CAD build for the part. Positions are in the model's coordinates, mm. A direction names the side the tool comes from. Round coordinates to 2 decimals unless told otherwise and drop trailing zeros. Order: outer loops, then holes, each group sorted by start corner. A loop starts at its lowest first (then second) coordinate and runs counter-clockwise, first axis right, second up. Notation, with made-up numbers: (27.5, -30) -> (52.5, -30) arc R16 ccw to (52.5, -24) -> close; hole circle Ø11 at (41.5, -6). An arc over 180 degrees is marked (long way). Return JSON: item names as keys, results as strings. Group by question number.
Q1. Flat gauge pins, fed straight in: pin 1 (1 mm diameter, centred on x = -29, y = -14.5, fed in from +Z); pin 2 (3 mm diameter, centred on x = -33, z = 2, fed in from -Y); pin 3 (3 mm diameter, centred on x = -46.5, y = -6.5, fed in from +Z). Where does each tip first touch, or does it go through?
Q2. Cut at A-A (z = 0). Write the cut outline in (x, y).
Q3. Mould opens along Z. For faces 4 (the flat face through (-70.245, -8.8, 9)), 5 (the cylindrical face through (-1.824, -60.029, -23.647)), 6 (the conical face through (10.1, 11.2, 36)) say: +Z half, -Z half, draft (parallel to the pull), parting line (faces both ways), or undercut.
Q4. Which spindle directions (+Z, -Z, +X, -X, +Y, -Y) get a long thin tool onto all of the face, cutting with end or side? Do faces 1 (the flat face through (-25.245, -36, 46)), 2 (the cylindrical face through (-1.824, 9.745, 23.647)), 3 (the flat face through (-42, -4.642, 0)). Say none if no direction does.
Q5. Probe line 1 along Y through (x, z) = (-50, 0); line 2 along X through (y, z) = (8, 7); line 3 along Y through (x, z) = (-15, 1). List the from-to ranges inside material, lowest first.
Q6. Cut at B-B (x = -11). Write the cut outline in (y, z).
Q7. Cut at C-C (x = -44.5). Write the cut outline in (y, z).
from build123d import *

# Parameters (mm, degrees)
CUT_EXTRUDE_1_DEPTH = 24.5
SKETCH_4_W          = 10
SKETCH_4_H          = 7.054294233
CUT_EXTRUDE_2_DEPTH = 109.585993287


with BuildPart() as part:
    # Эскиз1 → Повернуть1 (revolve)
    with BuildSketch(Plane.XY, mode=Mode.PRIVATE) as revolve_1_sk:
        with BuildLine():
            Line((-70.245087719, -6.642192982), (-70.245087719, 12.857807018))
            ThreePointArc((-70.245087719, 12.857807018), (-68.927068235, 16.039787533), (-65.745087719, 17.357807018))
            Line((-65.745087719, 17.357807018), (-29.745087719, 17.357807018))
            ThreePointArc((-29.745087719, 17.357807018), (-26.563107204, 18.675826502), (-25.245087719, 21.857807018))
            Line((-25.245087719, 21.857807018), (-25.245087719, 22.357807018))
            ThreePointArc((-25.245087719, 22.357807018), (-23.927068235, 25.539787533), (-20.745087719, 26.857807018))
            Line((-20.745087719, 26.857807018), (9.254912281, 26.857807018))
            Line((9.254912281, 26.857807018), (10.254912281, 25.857807018))
            Line((10.254912281, 25.857807018), (10.254912281, -6.642192982))
            Line((10.254912281, -6.642192982), (9.254912281, -7.642192982))
            Line((9.254912281, -7.642192982), (-69.245087719, -7.642192982))
            Line((-69.245087719, -7.642192982), (-70.245087719, -6.642192982))
        make_face()
    revolve(revolve_1_sk.sketch.rotate(Axis((-70.245087719, -25.142192982, 0), (1, 0, 0)), 90), axis=Axis((-70.245087719, -25.142192982, 0), (1, 0, 0)))

    # Эскиз3 → Вырез-Вытянуть1 (cut)
    with BuildSketch(Plane(origin=(10.254912281, 0, 0), x_dir=(0, 0, -1), z_dir=(1, 0, 0))):
        with BuildLine():
            ThreePointArc((-17.761912417, -50.549169727), (0, -93.142192982), (17.761912417, -50.549169727))
            ThreePointArc((17.761912417, -50.549169727), (21.920310217, -47.062503199), (25.406976744, -42.9041054))
            ThreePointArc((25.406976744, -42.9041054), (68, -25.142192982), (25.406976744, -7.380280565))
            ThreePointArc((25.406976744, -7.380280565), (21.920310217, -3.221882766), (17.761912417, 0.264783762))
            ThreePointArc((17.761912417, 0.264783762), (0, 42.857807018), (-17.761912417, 0.264783762))
            ThreePointArc((-17.761912417, 0.264783762), (-21.920310217, -3.221882766), (-25.406976744, -7.380280565))
            ThreePointArc((-25.406976744, -7.380280565), (-68, -25.142192982), (-25.406976744, -42.9041054))
            ThreePointArc((-25.406976744, -42.9041054), (-21.920310217, -47.062503199), (-17.761912417, -50.549169727))
        make_face()
    extrude(amount=-CUT_EXTRUDE_1_DEPTH, mode=Mode.SUBTRACT)

    # Эскиз4 → Вырез-Вытянуть2 (cut, through all)
    with BuildSketch(Plane(origin=(-14.245087719, 0, 0), x_dir=(0, 0, -1), z_dir=(1, 0, 0))):
        with Locations((0, -8.169340099)):
            Rectangle(SKETCH_4_W, SKETCH_4_H)
    extrude(amount=-CUT_EXTRUDE_2_DEPTH, mode=Mode.SUBTRACT)


solid = part.part
Solution:
{
 "1": {"pin 1": "stops at z = 41.38", "pin 2": "stops at y = -67.64", "pin 3": "stops at z = 38.89"},
 "2": {"outline": "(-70.25, -63.14) arc R4.5 ccw to (-65.75, -67.64) -> (-29.75, -67.64) arc R4.5 cw to (-25.25, -72.14) -> (-25.25, -72.64) arc R4.5 ccw to (-20.75, -77.14) -> (-14.25, -77.14) -> (-14.25, -42.64) -> (-69.25, -42.64) -> (-70.25, -43.64) -> close; (-70.25, -4.64) -> (-14.25, -4.64) -> (-14.25, 26.86) -> (-20.75, 26.86) arc R4.5 ccw to (-25.25, 22.36) -> (-25.25, 21.86) arc R4.5 cw to (-29.75, 17.36) -> (-65.75, 17.36) arc R4.5 ccw to (-70.25, 12.86) -> close"},
 "3": {"face 4": "draft", "face 5": "undercut", "face 6": "+Z half"},
 "4": {"face 1": "-X", "face 2": "+X", "face 3": "+X, -X"},
 "5": {"line 1": "y = -67.64 to -42.64, -4.64 to 17.36", "line 2": "x = -70.25 to -14.25", "line 3": "y = -77.13 to -42.61, -4.64 to 26.85"},
 "6": {"outline": "(-70.82, -24.86) arc R52 ccw to (-50, -45.67) arc R25 cw to (-42.9, -25.41) arc R31 cw to (-50.55, -17.76) arc R25 cw to start; (-70.82, 24.86) arc R25 cw to (-50.55, 17.76) arc R31 cw to (-42.9, 25.41) arc R25 cw to (-50, 45.67) arc R52 ccw to start; (-7.38, -25.41) arc R25 cw to (-0.29, -45.67) arc R52 ccw to (20.53, -24.86) arc R25 cw to (0.26, -17.76) arc R31 cw to start; (-7.38, 25.41) arc R31 cw to (0.26, 17.76) arc R25 cw to (20.53, 24.86) arc R52 ccw to (-0.29, 45.67) arc R25 cw to start"},
 "7": {"outline": "circle Ø85 at (-25.14, 0); hole (-8.37, -5) -> (-4.64, -5) -> (-4.64, 5) -> (-8.37, 5) arc R17.5 ccw (long way) to start"}
}
